The figure shows three views and two pictorial views of one solid part (mm, origin at its lowest corner). Answer the questions. A direction names the side the tool comes from. Give positions to 0.01 mm unless a question says otherwise; leave off trailing zeros. Write each loop counter-clockwise with the first axis right and the second up, starting at its lowest first coordinate (ties: lowest second). Pieces come first, ordered by that corner, then holes. Notation, with made-up numbers: (4.25, -24.5) - (62.25, -24.5) arc R7 ccw to (62.25, -18.5) - close; hole circle Ø6 at (25.25, 86). An arc over 180 degrees is marked (long way). One line per question, with ' | ' between items. Start each with the question number.
1. For the marked faces 1 and 2, determine the directions among +Z, -Z, +X, -X, +Y, -Y from which every point of the face is accessible in a straight line to the end or side of a thin tool.
2. A cutting plane is placed at D-D (z = 1.5). Determine the outline of the cut face in (x, y), then the cut area to 3 significant figures.
3. Given P1, Ø2.5, axis at x = 7.5, y = 7.5, coming from the +Z side; P2, Ø2, axis at y = 8.5, z = 5.5, coming from the -X side; P3, Ø3, axis at y = 15.5, z = 5.5, coming from the -X side, each flat-ended and moving along its own axis, determine where each tip first touches the part or whether it passes through.
4. Find the intervals of material crossed by L1, parallel to Y at x = 9, z = 5.75; L2, parallel to Z at x = 11, y = 11.5; L3, parallel to Z at x = 13.25, y = 16.25, in increasing order. Write a range as from..to.
5. A cutting plane is placed at A-A (x = 9). Determine the outline of the cut face in (y, z).
6. The mould has two halves that part along Y. Classify the marked faces 3, 4 and 5: +Y half, -Y half, draft (parallel to the pull), parting line (faces both ways), or undercut.
7. A cutting plane is placed at C-C (z = 3.75). Determine the outline of the cut face in (x, y), then the cut area to 3 significant figures.
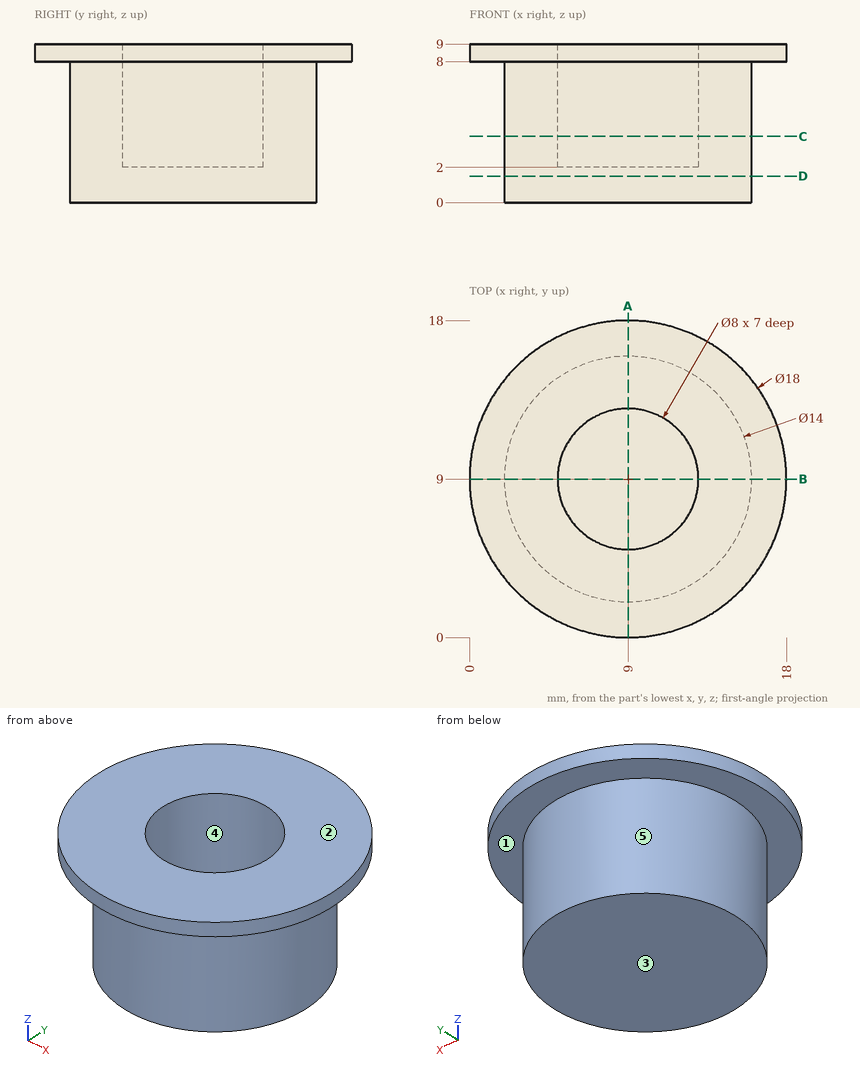
Determined:
1) face 1: -Z | face 2: +Z, +X, -X, +Y, -Y
2) outline: circle Ø14 at (9, 9) | area: 154 mm2
3) P1: z = 2 | P2: x = 2 | P3: x = 4.1
4) L1: 2..5, 13..16 | L2: 0..2 | L3: 8..9
5) outline: (0, 8) - (2, 8) - (2, 0) - (16, 0) - (16, 8) - (18, 8) - (18, 9) - (13, 9) - (13, 2) - (5, 2) - (5, 9) - (0, 9) - close
6) face 3: draft | face 4: undercut | face 5: parting line
7) outline: circle Ø14 at (9, 9); hole circle Ø8 at (9, 9) | area: 104 mm2
